Can you work these out from the model? Positions are in its coordinate system, mm. A direction names the side the tool comes from. Give positions to 0.01 mm unless a question says otherwise; leave off trailing zeros. Write each loop counter-clockwise with the first axis right and the second up, starting at its lowest first coordinate (ties: lowest second). Pieces come first, ordered by that corner, then holes.
from build123d import *

# Parameters (mm, degrees)
F0_W      = 50.8
F0_H      = 31.75
F1_DEPTH  = 69.85
F2_W      = 50.8
F2_H      = 38.1
F3_DEPTH  = 19.05
F5_DEPTH  = 19.05
F6_R      = 6.35
F8_DEPTH  = 25.4
F9_R      = 3.175
F10_DEPTH = 19.05


with BuildPart() as f1:
    # F0 (on Top) → F1 (new body)
    with BuildSketch(Plane.XY):
        with Locations((25.4, 15.875)):
            Rectangle(F0_W, F0_H)
    extrude(amount=F1_DEPTH)

    # F2 (on face) → F3 (cut)
    with BuildSketch(Plane.XZ):
        with Locations((25.4, 25.4)):
            Rectangle(F2_W, F2_H)
    extrude(amount=-F3_DEPTH, mode=Mode.SUBTRACT)

    # F4 (on face) → F5 (cut)
    with BuildSketch(Plane.XZ):
        with BuildLine():
            ThreePointArc((12.7, 57.15), (16.4197438789, 66.1302561211), (25.4, 69.85))
            Line((25.4, 69.85), (0, 69.85))
            Line((0, 69.85), (0, 44.45))
            Line((0, 44.45), (12.7, 44.45))
            Line((12.7, 44.45), (12.7, 57.15))
        make_face()
        with BuildLine():
            ThreePointArc((25.4, 69.85), (34.3802561211, 66.1302561211), (38.1, 57.15))
            Line((38.1, 57.15), (38.1, 44.45))
            Line((38.1, 44.45), (50.8, 44.45))
            Line((50.8, 44.45), (50.8, 69.85))
            Line((50.8, 69.85), (25.4, 69.85))
        make_face()
        with BuildLine():
            Line((38.1, 44.45), (38.1, 57.15))
            ThreePointArc((38.1, 57.15), (34.3802561211, 48.1697438789), (25.4, 44.45))
            Line((25.4, 44.45), (38.1, 44.45))
        make_face()
        with BuildLine():
            Line((12.7, 44.45), (25.4, 44.45))
            ThreePointArc((25.4, 44.45), (16.4197438789, 48.1697438789), (12.7, 57.15))
            Line((12.7, 57.15), (12.7, 44.45))
        make_face()
    extrude(amount=-F5_DEPTH, mode=Mode.SUBTRACT)

    # F7 (on face) + F6 (on face) → F8 (cut)
    with BuildSketch(Plane.XZ.offset(-19.05)):
        with BuildLine():
            ThreePointArc((25.4, 69.85), (34.3802561211, 66.1302561211), (38.1, 57.15))
            Line((38.1, 57.15), (38.1, 19.05))
            ThreePointArc((38.1, 19.05), (41.8197438789, 10.0697438789), (50.8, 6.35))
            Line((50.8, 6.35), (50.8, 69.85))
            Line((50.8, 69.85), (25.4, 69.85))
        make_face()
        with BuildLine():
            Line((12.7, 19.05), (12.7, 57.15))
            ThreePointArc((12.7, 57.15), (16.4197438789, 66.1302561211), (25.4, 69.85))
            Line((25.4, 69.85), (0, 69.85))
            Line((0, 69.85), (0, 6.35))
            ThreePointArc((0, 6.35), (8.9802561211, 10.0697438789), (12.7, 19.05))
        make_face()
    with BuildSketch(Plane.XZ):
        with Locations((25.4, 57.15)):
            Circle(F6_R)
    extrude(amount=-F8_DEPTH, mode=Mode.SUBTRACT)

    # F9 (on Top) → F10 (cut)
    with BuildSketch(Plane.XY):
        with Locations((41.275, 9.525)):
            Circle(F9_R)
        with Locations((9.525, 9.525)):
            Circle(F9_R)
    extrude(amount=F10_DEPTH, mode=Mode.SUBTRACT)


solid = f1.part
(1) Imagine slicing it at C-C, the plane x = 25.4. Write out the boundary of the cut face in (y, z), plus the area to 3 significant figures.
Returned:
outline: (0, 0) - (31.75, 0) - (31.75, 69.85) - (0, 69.85) - (0, 63.5) - (25.4, 63.5) - (25.4, 50.8) - (0, 50.8) - (0, 44.45) - (19.05, 44.45) - (19.05, 6.35) - (0, 6.35) - close
area: 1,170 mm2
(2) If I drill on L1, parallel to Z at x = 25.4, y = 17.75; L2, parallel to X at y = 15, z = 57; L3, parallel to Z at x = 29, y = 18, over which ranges is the centre line in solid material (lowest first)?
Returned:
L1: z = 0 to 6.35, 44.45 to 50.8, 63.5 to 69.85
L2: x = 12.7 to 19.05, 31.75 to 38.1
L3: z = 0 to 6.35, 44.97 to 51.92, 62.38 to 69.33
(3) Imagine slicing it at D-D, the plane z = 53.5. Write out the boundary of the cut face in (x, y).
Returned:
outline: (12.7, 19.05) - (13.24, 19.05) - (13.24, 0) - (20.2, 0) - (20.2, 25.4) - (30.6, 25.4) - (30.6, 0) - (37.56, 0) - (37.56, 19.05) - (38.1, 19.05) - (38.1, 31.75) - (12.7, 31.75) - close
(4) Imagine slicing it at A-A, the plane y = 29.5. Write out the boundary of the cut face in (x, z), plus the area to 3 significant figures.
Returned:
outline: (0, 0) - (50.8, 0) - (50.8, 6.35) arc R12.7 cw to (38.1, 19.05) - (38.1, 57.15) arc R12.7 ccw to (12.7, 57.15) - (12.7, 19.05) arc R12.7 cw to (0, 6.35) - close
area: 1,940 mm2
(5) For faces 4 (the face through (12.7, 25, 38)), 5 (the face through (27.053, 12.125, 69.742)), 6 (the face through (25, 9, 6.35)), 7 (the face through (0, 16, 3)), which set-ups out of +Z, -Z, +X, -X, +Y, -Y let a thin tool reach every point of the face, with its end or its side?
Returned:
face 4: +Z, -X, +Y, -Y
face 5: -Y
face 6: +X, -X, -Y
face 7: +Z, -Z, -X, +Y, -Y
(6) Imagine slicing it at B-B, the plane x = 41.5. Write out the boundary of the cut face in (y, z).
Returned:
outline: (0, 0) - (6.36, 0) - (6.36, 6.35) - (0, 6.35) - close; (12.69, 0) - (31.75, 0) - (31.75, 10.4) - (19.05, 10.4) - (19.05, 6.35) - (12.69, 6.35) - close
(7) Will these pins go through, and if not, where does the flat tip stop? P1, Ø3, axis at x = 13, z = 29.5, coming from the -Y side; P2, Ø3, axis at y = 23.5, z = 37.5, coming from the -X side; P3, Ø4, axis at x = 26.5, z = 56.5, coming from the -Y side.
Returned:
P1: stops at y = 19.05
P2: stops at x = 12.7
P3: stops at y = 25.4
(8) If we mould it in two halves opening along X, with no side actions, what happens to faces 1 (the face through (24.02, 12.52, 50.95)), 2 (the face through (38.1, 25, 38)), 3 (the face through (25, 31.75, 27))? For each: +X half, -X half, draft (parallel to the pull), parting line (faces both ways), or undercut.
Returned:
face 1: undercut
face 2: +X half
face 3: draft
